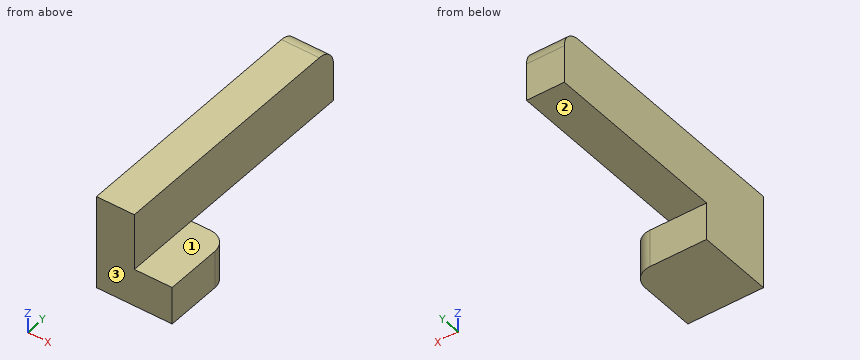
from build123d import *

# Parameters (mm, degrees)
SKETCH1_W           = 20
SKETCH1_H           = 140
BOSS_EXTRUDE1_DEPTH = 30
SKETCH2_W           = 40
SKETCH2_H           = 40
BOSS_EXTRUDE2_DEPTH = 20
FILLET1_R           = 10


with BuildPart() as part:
    # Sketch1 → Boss-Extrude1 (new body)
    with BuildSketch(Plane.XY):
        with Locations((-20, -70)):
            Rectangle(SKETCH1_W, SKETCH1_H)
    extrude(amount=BOSS_EXTRUDE1_DEPTH)

    # Sketch2 → Boss-Extrude2 (add)
    with BuildSketch(Plane.XY):
        with Locations((-10, -120)):
            Rectangle(SKETCH2_W, SKETCH2_H)
    extrude(amount=-BOSS_EXTRUDE2_DEPTH)

    # Fillet1
    fillet1_edges = [part.edges().sort_by_distance(p)[0] for p in [
        (10, -100, -10),
        (-20, 0, 30),
    ]]
    fillet(fillet1_edges, radius=FILLET1_R)


solid = part.part
CAD build for the part. Positions are in the model's coordinates, mm. Face numbers are marked on the shaded views. A direction names the side the tool comes from. Round coordinates to 2 decimals unless told otherwise and drop trailing zeros. Order: outer loops, then holes, each group sorted by start corner. A loop starts at its lowest first (then second) coordinate and runs counter-clockwise, first axis right, second up. Notation, with made-up numbers: (77.25, 11) -> (121.25, 11) arc R26 ccw to (121.25, 49) -> close; hole circle Ø4 at (77, -7). An arc over 180 degrees is marked (long way). Write item = value, one per line. Start each with the question number.
(1) Cut at A-A, the plane z = -13. List the corners of the cut face in (x, y), then the cut area to 3 significant figures.
(2) Probe line 1 (Z direction, x = -20, y = -44.5); line 2 (X direction, y = -80.5, z = 4.5); line 3 (Y direction, x = -0.5, z = -15). List the from-to ranges inside material, lowest first. Write a range as [from, to].
(3) Cut at D-D, the plane y = -61.5. List the corners of the cut face in (x, z), then the cut area to 3 significant figures.
(4) Pin check, flat tips, straight feed: P1, Ø10, axis at x = -17.5, z = -14, coming from the +Y side; P2, Ø2, axis at x = -21, y = -97, coming from the -Z side; P3, Ø10, axis at x = 2, y = -110.5, coming from the +Z side. Stop position of each tip, or through.
(5) Which spindle directions (+Z, -Z, +X, -X, +Y, -Y) get a long thin tool onto all of the face, cutting with end or side? Do the marked faces 1, 2 and 3. Say none if no direction does.
(6) Cut at C-C, the plane x = -19. List the corners of the cut face in (y, z).
(7) Cut at B-B, the plane y = -130.5. List the corners of the cut face in (x, z).
Model answer:
q1.outline = (-30, -140) -> (10, -140) -> (10, -110) arc R10 ccw to (0, -100) -> (-30, -100) -> close
q1.area = 1,580 mm2
q2.line_1 = [0, 30]
q2.line_2 = [-30, -10]
q2.line_3 = [-140, -100]
q3.outline = (-30, 0) -> (-10, 0) -> (-10, 30) -> (-30, 30) -> close
q3.area = 600 mm2
q4.P1 = -100
q4.P2 = 0
q4.P3 = 0
q5.face_1 = +Z, +X, +Y, -Y
q5.face_2 = -Z, +X, -X, +Y
q5.face_3 = +Z, -Z, +X, -X, -Y
q6.outline = (-140, -20) -> (-100, -20) -> (-100, 0) -> (0, 0) -> (0, 20) arc R10 ccw to (-10, 30) -> (-140, 30) -> close
q7.outline = (-30, -20) -> (10, -20) -> (10, 0) -> (-10, 0) -> (-10, 30) -> (-30, 30) -> close
